Design review of the part built by this model. Coordinates are the model's own, in mm. A direction names the side the tool comes from. Coordinates: 2 decimals unless noted, no trailing zeros. Loops run counter-clockwise (first coordinate to the right, second up) from the corner with the lowest first, then second, coordinate; pieces in that order, holes last. Notation, with made-up numbers: (32, 87) -> (63, 87) arc R25 ccw to (63, 113) -> close; hole circle Ø5 at (72.25, 81). An arc over 180 degrees is marked (long way). Use CSV: the item, a comma, the result in double quotes.
```python
from build123d import *

# Parameters (mm, degrees)
PAD003_DEPTH    = 2
SKETCH009_R     = 3
SKETCH009_R_2   = 2.5
PAD004_DEPTH    = 4.75
SKETCH010_R     = 1.5
SKETCH010_R_2   = 1.4
SKETCH010_R_3   = 1.12
POCKET001_DEPTH = 4.75
PAD006_DEPTH    = 35
SKETCH017_R     = 1.12
POCKET007_DEPTH = 4.75
POCKET008_DEPTH = 35


with BuildPart() as part:
    # Sketch007 (on Origin) → Pad003 (new body)
    with BuildSketch(Plane.XZ.offset(-10.46)):
        Polygon((-35.76, 31.05), (1.64, 31.05), (1.64, 36.05), (15.64, 36.05), (15.64, 31.05), (35.24, 31.05), (35.24, -40.03), (-35.76, -40.03), align=None)
    extrude(amount=PAD003_DEPTH)

    # Sketch009 → Pad004 (join)
    with BuildSketch(Plane(origin=(0, 8.5, 0), x_dir=(1, 0, 0), z_dir=(0, 1, 0))):
        with Locations((-4.91, 33.77)):
            Circle(SKETCH009_R)
        with Locations((-29.29, 33.77)):
            Circle(SKETCH009_R)
        with Locations((-29.29, 7.54)):
            Circle(SKETCH009_R)
        with Locations((-4.91, 7.54)):
            Circle(SKETCH009_R)
        with Locations((30.36, 33.28)):
            Circle(SKETCH009_R_2)
        with Locations((18.93, 33.28)):
            Circle(SKETCH009_R_2)
        with Locations((18.55, 16.9)):
            Circle(SKETCH009_R_2)
        with Locations((30.74, 16.9)):
            Circle(SKETCH009_R_2)
        with Locations((28.74, -24.55)):
            Circle(SKETCH009_R)
        with Locations((-29.26, -24.55)):
            Circle(SKETCH009_R)
        with Locations((-29.26, -1.55)):
            Circle(SKETCH009_R)
        with Locations((28.74, -1.55)):
            Circle(SKETCH009_R)
    extrude(amount=-PAD004_DEPTH)

    # Sketch010 (on Face33 of Pad004) → Pocket001 (cut)
    with BuildSketch(Plane.XZ.offset(-3.75)):
        with Locations((-29.26, 24.55)):
            Circle(SKETCH010_R)
        with Locations((-29.26, 1.55)):
            Circle(SKETCH010_R)
        with Locations((28.74, 1.55)):
            Circle(SKETCH010_R)
        with Locations((28.74, 24.55)):
            Circle(SKETCH010_R)
        with Locations((-29.29, -7.54)):
            Circle(SKETCH010_R_2)
        with Locations((-4.91, -7.54)):
            Circle(SKETCH010_R_2)
        with Locations((-4.91, -33.77)):
            Circle(SKETCH010_R_2)
        with Locations((-29.29, -33.77)):
            Circle(SKETCH010_R_2)
        with Locations((18.55, -16.9)):
            Circle(SKETCH010_R_3)
        with Locations((30.74, -16.9)):
            Circle(SKETCH010_R_3)
        with Locations((30.36, -33.28)):
            Circle(SKETCH010_R_3)
        with Locations((18.93, -33.28)):
            Circle(SKETCH010_R_3)
    extrude(amount=-POCKET001_DEPTH, mode=Mode.SUBTRACT)

    # Sketch016 (on DatumPlane) → Pad006 (join)
    with BuildSketch(Plane(origin=(0, 10.46, -38.03), x_dir=(1, 0, 0), z_dir=(0, 0, -1))):
        Polygon((-33.76, 2), (-32.76, 4.5), (-33.56, 6.5), (-33.26, 7), (-32.26, 7), (-32.26, 2), align=None)
        Polygon((33.24, 2), (32.24, 4.5), (33.04, 6.5), (32.74, 7), (31.74, 7), (31.74, 2), align=None)
    extrude(amount=-PAD006_DEPTH)

    # Sketch017 (on Face46 of Pad006) → Pocket007 (cut, symmetric)
    with BuildSketch(Plane.XZ.offset(-3.75)):
        with Locations((30.74, -16.9)):
            Circle(SKETCH017_R)
    extrude(amount=POCKET007_DEPTH, both=True, mode=Mode.SUBTRACT)

    # Sketch018 (on Face32 of Pocket007) → Pocket008 (cut)
    with BuildSketch(Plane(origin=(0, 10.46, -38.03), x_dir=(1, 0, 0), z_dir=(0, 0, -1))):
        Polygon((35.24, 2), (33.24, 2), (32.24, 4.5), (33.04, 6.5), (32.74, 7), (35.24, 7), align=None)
    extrude(amount=-POCKET008_DEPTH, mode=Mode.SUBTRACT)


solid = part.part
```
Item 1: Add section C-C (z = -27.5). Give the boundary of the cut face in (x, y), then the cut area to 3 significant figures.
Checked values:
outline,"(-35.76, 8.46) -> (-33.76, 8.46) -> (-32.76, 5.96) -> (-33.56, 3.96) -> (-33.26, 3.46) -> (-32.26, 3.46) -> (-32.26, 8.46) -> (31.74, 8.46) -> (31.74, 3.46) -> (32.74, 3.46) -> (33.04, 3.96) -> (32.24, 5.96) -> (33.24, 8.46) -> (35.24, 8.46) -> (35.24, 10.46) -> (-35.76, 10.46) -> close"
area,"152 mm^2"
Item 2: Machinability: for faces 1 (the face through (-33.154, 4.974, -20.775)), 2 (the face through (21.24, 6.14, -32.32)), 3 (the face through (15.64, 9, 34)), 4 (the face through (20, 3.75, -16)), which of the approach directions +Z, -Z, +X, -X, +Y, -Y give a long, thin tool a straight path to every point of the face, cutting with its end or side? Answer none if there is none.
Checked values:
face 1,"+Z, -Z, -X"
face 2,"-Y"
face 3,"+Z, +X, +Y, -Y"
face 4,"+Z, -Z, -Y"
Item 3: Draft analysis for pull direction Z (two halves, no side actions). For faces 5 (the face through (31.74, 6, -10)), 6 (the face through (35.24, 9, -4)), state which applies: pulls with the +Z half, pulls with the -Z half, needs draft (parallel to the pull), parting line crosses it, or undercut.
Checked values:
face 5,"undercut"
face 6,"needs draft"
Item 4: Clearance check with flat-ended pins moving along their axes: pin 1 (5 mm diameter, centred on x = 28.74, z = 24.55, fed in from -Y); pin 2 (10 mm diameter, centred on x = -6.5, z = 9.5, fed in from -Y); pin 3 (1 mm diameter, centred on x = -24.5, y = 10, fed in from +Z); pin 4 (0.5 mm diameter, centred on x = 33, y = 7, fed in from +Z). State where each tip first meets the part, or that it passes through.
Checked values:
pin 1,"y = 3.75"
pin 2,"y = 8.46"
pin 3,"z = 31.05"
pin 4,"through"
Item 5: Add section A-A (z = 1.55). Give the boundary of the cut face in (x, y).
Checked values:
outline,"(-35.76, 8.46) -> (-32.26, 8.46) -> (-32.26, 3.75) -> (-30.76, 3.75) -> (-30.76, 8.5) -> (-27.76, 8.5) -> (-27.76, 3.75) -> (-26.26, 3.75) -> (-26.26, 8.46) -> (25.74, 8.46) -> (25.74, 3.75) -> (27.24, 3.75) -> (27.24, 8.5) -> (30.24, 8.5) -> (30.24, 3.75) -> (31.74, 3.75) -> (31.74, 8.46) -> (35.24, 8.46) -> (35.24, 10.46) -> (-35.76, 10.46) -> close"
Item 6: Add section D-D (z = 18.5). Give the boundary of the cut face in (x, y), then the cut area to 3 significant figures.
Checked values:
outline,"(-35.76, 8.46) -> (35.24, 8.46) -> (35.24, 10.46) -> (-35.76, 10.46) -> close"
area,"142 mm^2"
Item 7: Add section B-B (y = 7.5). State how many separate pieces and enclosed holes the cut face has, then the cut area to 3 significant figures.
Checked values:
separate pieces,"10"
enclosed holes,"12"
area,"306 mm^2"
Item 8: To check wall thickness, follow line 1 along Z through (x, y) = (-4.91, 5.8); line 2 along Z through (x, y) = (-4, 5); line 3 along Z through (x, y) = (30.74, 5.3). State the ranges of each line that lie inside material, in increasing order.
Checked values:
line 1,"-36.77 to -35.17, -32.37 to -30.77, -10.54 to -8.94, -6.14 to -4.54"
line 2,"-36.63 to -34.83, -32.71 to -30.91, -10.4 to -8.6, -6.48 to -4.68"
line 3,"-35.75 to -34.33, -32.23 to -30.81, -19.4 to -18.02, -15.78 to -14.4, -0.69 to 3.79, 22.31 to 26.79"
